Model file for the job. Use its own axes, mm. A direction names the side the tool comes from. Round coordinates to 2 decimals unless told otherwise and drop trailing zeros. Write each loop counter-clockwise with the first axis right and the second up, starting at its lowest first coordinate (ties: lowest second). Pieces come first, ordered by that corner, then holes.
```python
from build123d import *

# Parameters (mm, degrees)
BOSS_EXTRU_1_DEPTH           = 10
ENL_V_MAT_EXTRU_1_DEPTH      = 66.048059156
ENL_V_MAT_EXTRU_1_DEPTH_BACK = 66.048059156


with BuildPart() as part:
    # Esquisse1 → Boss.-Extru.1 (new body)
    with BuildSketch(Plane(origin=(0, 0, 0), x_dir=(1, 0, 0), z_dir=(0, 1, 0))):
        with BuildLine():
            Line((-15, 62.5), (-15, 50))
            ThreePointArc((-15, 50), (-7.928932188, 47.071067812), (-5, 40))
            Line((-5, 40), (-5, -40))
            ThreePointArc((-5, -40), (-7.928932188, -47.071067812), (-15, -50))
            Line((-15, -50), (-15, -62.5))
            ThreePointArc((-15, -62.5), (0, -54.472243623), (15, -62.5))
            Line((15, -62.5), (15, -50))
            ThreePointArc((15, -50), (7.928932188, -47.071067812), (5, -40))
            Line((5, -40), (5, 40))
            ThreePointArc((5, 40), (7.928932188, 47.071067812), (15, 50))
            Line((15, 50), (15, 62.5))
            ThreePointArc((15, 62.5), (0, 54.472243623), (-15, 62.5))
        make_face()
    extrude(amount=BOSS_EXTRU_1_DEPTH)

    # Esquisse2 → Enlèv. mat.-Extru.1 (cut, two sides: drawn at the far end of the back side and taken through both)
    with BuildSketch(Plane.XY.offset(-ENL_V_MAT_EXTRU_1_DEPTH_BACK)):
        with BuildLine():
            ThreePointArc((-15, 10), (-8.117941502, 5.401555527), (0, 3.786796564))
            Line((0, 3.786796564), (0, 10))
            Line((0, 10), (-15, 10))
        make_face()
        with BuildLine():
            Line((0, 10), (0, 3.786796564))
            ThreePointArc((0, 3.786796564), (8.117941502, 5.401555527), (15, 10))
            Line((15, 10), (0, 10))
        make_face()
        with BuildLine():
            ThreePointArc((-15, 10), (-8.117941502, 5.401555527), (0, 3.786796564))
            Line((0, 3.786796564), (0, 10))
            Line((0, 10), (-15, 10))
        make_face()
        with BuildLine():
            Line((0, 10), (0, 3.786796564))
            ThreePointArc((0, 3.786796564), (8.117941502, 5.401555527), (15, 10))
            Line((15, 10), (0, 10))
        make_face()
    extrude(amount=ENL_V_MAT_EXTRU_1_DEPTH + ENL_V_MAT_EXTRU_1_DEPTH_BACK, mode=Mode.SUBTRACT)


solid = part.part
```
1) Which spindle directions (+Z, -Z, +X, -X, +Y, -Y) get a long thin tool onto all of the face, cutting with end or side? Do faces 5 (the face through (0, 0, -1)), 6 (the face through (9, 3, 48)), 7 (the face through (-9, 3, -48)). Say none if no direction does.
2) Pull direction X, two halves, no side cores. Call faces 1 (the face through (15, 5, -56)), 2 (the face through (0.248, 2.708, -54.474)), 3 (the face through (-5, 2, -1)), 4 (the face through (-0.248, 2.708, 54.474)): released by +X, released by -X, zero draft, split by the parting line, or undercut.
3) Cut at A-A on y = 5.5. List the corners of the cut face in (x, z), and give its area (3 significant figures).
4) Cut at B-B on x = -6.5. List the corners of the cut face in (y, z), and give its area (3 significant figures).
5) Cut at D-D on z = 44.5. List the corners of the cut face in (x, y), and give its area (3 significant figures).
6) Flat gauge pins, fed straight in: pin 1 Ø8 at (x, z) = (11.5, 19.5) entering from -Y; pin 2 Ø3.5 at (y, z) = (2, 8.5) entering from +X; pin 3 Ø6 at (x, y) = (11, 5.5) entering from -Z; pin 4 Ø3 at (x, z) = (-0.5, -29.5) entering from +Y. Where does each tip first touch, or does it go through?
7) Wall check: probe 1 along X at (y, z) = (2.25, 13); probe 2 along Z at (x, y) = (10.5, 2); probe 3 along X at (y, z) = (9, 56). Give the ranges that are in metal, low to high.
8) Cut at C-C on z = -19.5. List the corners of the cut face in (x, y), and give its area (3 significant figures).
Result sheet:
1. face 5: +Z, -Z, +X, -X, -Y
1. face 6: +X, +Y, -Y
1. face 7: -X, +Y, -Y
2. face 1: released by +X
2. face 2: undercut
2. face 3: released by -X
2. face 4: undercut
3. outline: (-15, -62.5) arc R18.03 cw to (-8.35, -56.52) - (-8.35, -47.47) arc R10 cw to (-15, -50) - close; (-15, 50) arc R10 cw to (-8.35, 47.47) - (-8.35, 56.52) arc R18.03 cw to (-15, 62.5) - close; (8.35, -56.52) arc R18.03 cw to (15, -62.5) - (15, -50) arc R10 cw to (8.35, -47.47) - close; (8.35, 47.47) arc R10 cw to (15, 50) - (15, 62.5) arc R18.03 cw to (8.35, 56.52) - close
3. area: 261 mm2
4. outline: (0, -55.68) - (4.81, -55.68) - (4.81, -45.27) - (0, -45.27) - close; (0, 45.27) - (4.81, 45.27) - (4.81, 55.68) - (0, 55.68) - close
4. area: 100 mm2
5. outline: (-6.07, 0) - (6.07, 0) - (6.07, 4.67) arc R21.21 cw to (-6.07, 4.67) - close
5. area: 49.5 mm2
6. pin 1: passes through
6. pin 2: stops at x = 5
6. pin 3: stops at z = -61.14
6. pin 4: stops at y = 3.88
7. probe 1: x = -5 to 5
7. probe 2: z = -57.85 to -48.93, 48.93 to 57.85
7. probe 3: x = -15 to -13.93, 13.93 to 15
8. outline: (-5, 0) - (5, 0) - (5, 4.38) arc R21.21 cw to (-5, 4.38) - close
8. area: 39.8 mm2
